from build123d import *

# Parameters (mm, degrees)
SKETCH1_W           = 406.4
SKETCH1_H           = 101.6
BOSS_EXTRUDE1_DEPTH = 17.9832
SKETCH2_W           = 88.9
SKETCH2_H           = 38.1
CUT_EXTRUDE1_DEPTH  = 228.895141419
FILLET1_R           = 16.51


with BuildPart() as part:
    # Sketch1 → Boss-Extrude1 (new body)
    with BuildSketch(Plane.XY):
        with Locations((0, 50.8)):
            Rectangle(SKETCH1_W, SKETCH1_H)
    extrude(amount=BOSS_EXTRUDE1_DEPTH)

    # Sketch2 → Cut-Extrude1 (cut, through all)
    with BuildSketch(Plane.XY.offset(17.9832)):
        with Locations((-158.75, 82.55)):
            Rectangle(SKETCH2_W, SKETCH2_H)
        with Locations((158.75, 82.55)):
            Rectangle(SKETCH2_W, SKETCH2_H)
    extrude(amount=-CUT_EXTRUDE1_DEPTH, mode=Mode.SUBTRACT)

    # Fillet1
    fillet1_edges = [part.edges().sort_by_distance(p)[0] for p in [
        (-203.2, 63.5, 8.9916),
        (-114.3, 101.6, 8.9916),
        (-114.3, 63.5, 8.9916),
        (203.2, 63.5, 8.9916),
        (114.3, 63.5, 8.9916),
        (114.3, 101.6, 8.9916),
    ]]
    fillet(fillet1_edges, radius=FILLET1_R)


solid = part.part
Work out the finished part from the listing and answer in its coordinate system (mm). A direction names the side the tool comes from. Round coordinates to 2 decimals unless told otherwise and drop trailing zeros. Write each loop counter-clockwise with the first axis right and the second up, starting at its lowest first coordinate (ties: lowest second). Pieces come first, ordered by that corner, then holes. Notation, with made-up numbers: M 31,73.25 L 56,73.25 A33 cw 56,105.25 Z; hole C -21.75,50.5 d9. An arc over 180 degrees is marked long. Use a Markdown table: item, result.
1) Determine the mould class of faces 1 (the face through (109.34, 96.89, 8.87)), 2 (the face through (-3, 0, 9)), 3 (the face through (-198.49, 58.54, 8.87)) for opening direction X: pulls with the +X half, pulls with the -X half, needs draft (parallel to the pull), parting line crosses it, or undercut.
Taken from the geometry:
| item | result |
|---|---|
| face 1 | pulls with the +X half |
| face 2 | needs draft |
| face 3 | pulls with the -X half |
2) Which of the six approach directions +Z, -Z, +X, -X, +Y, -Y give full straight-line access (tool end or side, diameter ignored) to faces 4 (the face through (158, 63.5, 9)), 5 (the face through (-159, 63.5, 9)), 6 (the face through (-203.2, 23, 9))?
Taken from the geometry:
| item | result |
|---|---|
| face 4 | +Z, -Z, +X, +Y |
| face 5 | +Z, -Z, -X, +Y |
| face 6 | +Z, -Z, -X, +Y, -Y |
3) Consider line 1 (X direction, y = 80, z = 9.25); line 2 (X direction, y = 48, z = 9); line 3 (Y direction, x = -140.5, z = 9.5). Determine where each line is inside the solid, lowest interval first. Write a range as [from, to].
Taken from the geometry:
| item | result |
|---|---|
| line 1 | x = [-114.3, 114.3] |
| line 2 | x = [-203.17, 203.17] |
| line 3 | y = [0, 63.5] |
4) The part is cut by section A-A on z = 14.5. Give the vertices of the cut face in (x, y).
Taken from the geometry:
| item | result |
|---|---|
| outline | M -203.2,0 L 203.2,0 L 203.2,46.99 A16.51 ccw 186.69,63.5 L 130.81,63.5 A16.51 cw 114.3,80.01 L 114.3,85.09 A16.51 ccw 97.79,101.6 L -97.79,101.6 A16.51 ccw -114.3,85.09 L -114.3,80.01 A16.51 cw -130.81,63.5 L -186.69,63.5 A16.51 ccw -203.2,46.99 Z |
5) The part is cut by section B-B on y = 75.5. Give the vertices of the cut face in (x, z), plus the area to 3 significant figures.
Taken from the geometry:
| item | result |
|---|---|
| outline | M -114.93,0 L 114.93,0 L 114.93,17.98 L -114.93,17.98 Z |
| area | 4,130 mm2 |
6) Flat-ended cylindrical pins translate along their axes: pin 1 (1.5 mm diameter, centred on y = 82, z = 5, fed in from +X); pin 2 (5 mm diameter, centred on x = 142.5, z = 2, fed in from +Y); pin 3 (3 mm diameter, centred on y = 81.5, z = 13.5, fed in from -X). Find the tip coordinate at first contact, or state that the pin passes through.
Taken from the geometry:
| item | result |
|---|---|
| pin 1 | stops at x = 114.3 |
| pin 2 | stops at y = 63.5 |
| pin 3 | stops at x = -114.3 |
7) The part is cut by section C-C on x = 122.5. Give the vertices of the cut face in (y, z).
Taken from the geometry:
| item | result |
|---|---|
| outline | M 0,0 L 65.74,0 L 65.74,17.98 L 0,17.98 Z |
